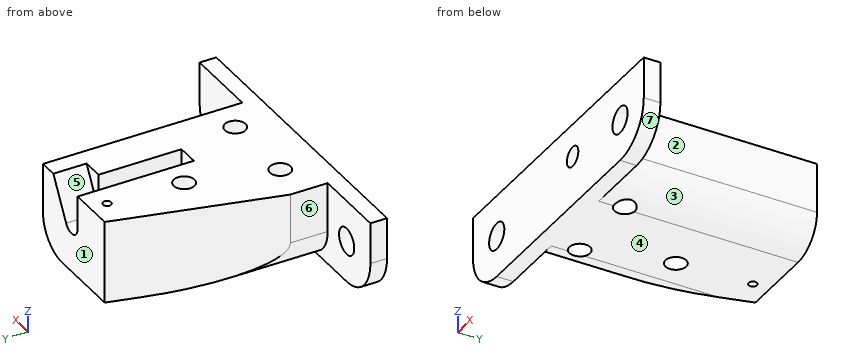
```python
from build123d import *

# Parameters (mm, degrees)
SKETCH1_R           = 1.6
BOSS_EXTRUDE1_DEPTH = 2
BOSS_EXTRUDE2_DEPTH = 26
CUT_EXTRUDE1_REACH  = 28
SKETCH3_R           = 1.2
CUT_EXTRUDE2_DEPTH  = 4
CUT_EXTRUDE3_DEPTH  = 14
CUT_EXTRUDE4_REACH  = 12
SKETCH6_R           = 0.5
SKETCH6_R_2         = 1.25


with BuildPart() as part:
    # Sketch1 → Boss-Extrude1 (new body)
    with BuildSketch(Plane(origin=(0, 0, 0), x_dir=(1, 0, 0), z_dir=(0, 1, 0))):
        with BuildLine():
            Line((0, 0), (36, 0))
            Line((36, 0), (36, 5))
            ThreePointArc((36, 5), (34.535533906, 8.535533906), (31, 10))
            Line((31, 10), (27, 10))
            Line((27, 10), (9, 10))
            Line((9, 10), (5, 10))
            ThreePointArc((5, 10), (1.464466094, 8.535533906), (0, 5))
            Line((0, 5), (0, 0))
        make_face()
        with Locations((5, 5)):
            Circle(SKETCH1_R, mode=Mode.SUBTRACT)
        with Locations((31, 5)):
            Circle(SKETCH1_R, mode=Mode.SUBTRACT)
    extrude(amount=BOSS_EXTRUDE1_DEPTH)

    # Sketch2 → Boss-Extrude2 (add)
    with BuildSketch(Plane(origin=(0, 0, 0), x_dir=(1, 0, 0), z_dir=(0, 1, 0))):
        with BuildLine():
            Line((27, 0), (27, 6))
            ThreePointArc((27, 6), (25.828427125, 8.828427125), (23, 10))
            Line((23, 10), (13, 10))
            ThreePointArc((13, 10), (10.171572875, 8.828427125), (9, 6))
            Line((9, 6), (9, 0))
            Line((9, 0), (27, 0))
        make_face()
    extrude(amount=BOSS_EXTRUDE2_DEPTH)

    # Sketch3 → Cut-Extrude1 (cut, up to next)
    with BuildSketch(Plane(origin=(0, 26, 0), x_dir=(1, 0, 0), z_dir=(0, 1, 0)), mode=Mode.PRIVATE) as cut_extrude1_sk1:
        with Locations((21, 4)):
            Circle(SKETCH3_R)
    cut_extrude1_tool1 = extrude(cut_extrude1_sk1.sketch, amount=-CUT_EXTRUDE1_REACH, mode=Mode.PRIVATE) & part.part
    add(cut_extrude1_tool1.solids().sort_by_distance((21, 26, -4))[0], mode=Mode.SUBTRACT)

    # Sketch4 → Cut-Extrude2 (cut)
    with BuildSketch(Plane(origin=(0, 26, 0), x_dir=(1, 0, 0), z_dir=(0, 1, 0))):
        with BuildLine():
            Line((22.125833025, 4.65), (24.810511777, 0))
            Line((24.810511777, 0), (19.7, 0))
            Line((19.7, 0), (19.7, 4))
            ThreePointArc((19.7, 4), (20.663535241, 5.255703574), (22.125833025, 4.65))
        make_face()
    extrude(amount=-CUT_EXTRUDE2_DEPTH, mode=Mode.SUBTRACT)

    # Sketch5 → Cut-Extrude3 (cut)
    with BuildSketch(Plane(origin=(0, 26, 0), x_dir=(1, 0, 0), z_dir=(0, 1, 0))):
        with BuildLine():
            Line((19.7, 4), (19.7, 0))
            Line((19.7, 0), (22.3, 0))
            Line((22.3, 0), (22.3, 4))
            ThreePointArc((22.3, 4), (21, 5.3), (19.7, 4))
        make_face()
    extrude(amount=-CUT_EXTRUDE3_DEPTH, mode=Mode.SUBTRACT)

    # Sketch6 → Cut-Extrude4 (cut, up to next)
    with BuildSketch(Plane.XY, mode=Mode.PRIVATE) as cut_extrude4_sk1:
        with Locations((17, 24)):
            Circle(SKETCH6_R)
    cut_extrude4_tool1 = extrude(cut_extrude4_sk1.sketch, amount=-CUT_EXTRUDE4_REACH, mode=Mode.PRIVATE) & part.part
    add(cut_extrude4_tool1.solids().sort_by_distance((17, 24, 0))[0], mode=Mode.SUBTRACT)
    # Sketch6 → Cut-Extrude4 (cut, up to next)
    with BuildSketch(Plane.XY, mode=Mode.PRIVATE) as cut_extrude4_sk2:
        with Locations((16.5, 15)):
            Circle(SKETCH6_R_2)
    cut_extrude4_tool2 = extrude(cut_extrude4_sk2.sketch, amount=-CUT_EXTRUDE4_REACH, mode=Mode.PRIVATE) & part.part
    add(cut_extrude4_tool2.solids().sort_by_distance((16.5, 15, 0))[0], mode=Mode.SUBTRACT)
    # Sketch6 → Cut-Extrude4 (cut, up to next)
    with BuildSketch(Plane.XY, mode=Mode.PRIVATE) as cut_extrude4_sk3:
        with Locations((13.75, 5)):
            Circle(SKETCH6_R_2)
    cut_extrude4_tool3 = extrude(cut_extrude4_sk3.sketch, amount=-CUT_EXTRUDE4_REACH, mode=Mode.PRIVATE) & part.part
    add(cut_extrude4_tool3.solids().sort_by_distance((13.75, 5, 0))[0], mode=Mode.SUBTRACT)
    # Sketch6 → Cut-Extrude4 (cut, up to next)
    with BuildSketch(Plane.XY, mode=Mode.PRIVATE) as cut_extrude4_sk4:
        with Locations((23.25, 5)):
            Circle(SKETCH6_R_2)
    cut_extrude4_tool4 = extrude(cut_extrude4_sk4.sketch, amount=-CUT_EXTRUDE4_REACH, mode=Mode.PRIVATE) & part.part
    add(cut_extrude4_tool4.solids().sort_by_distance((23.25, 5, 0))[0], mode=Mode.SUBTRACT)
    # Sketch6 → Cut-Extrude4 (cut, up to next)
    with BuildSketch(Plane.XY, mode=Mode.PRIVATE) as cut_extrude4_sk5:
        Polygon((9, 6.5), (14, 26), (9, 26), align=None)
    cut_extrude4_tool5 = extrude(cut_extrude4_sk5.sketch, amount=-CUT_EXTRUDE4_REACH, mode=Mode.PRIVATE) & part.part
    add(cut_extrude4_tool5.solids().sort_by_distance((10.666667, 19.5, 0))[0], mode=Mode.SUBTRACT)


solid = part.part
```
For this review, take the finished solid that the model builds, in its own axes (mm). Face numbers are marked on the shaded views. A direction names the side the tool comes from. Round coordinates to 2 decimals unless told otherwise and drop trailing zeros. Order: outer loops, then holes, each group sorted by start corner. A loop starts at its lowest first (then second) coordinate and runs counter-clockwise, first axis right, second up. Notation, with made-up numbers: (74, 31) -> (85, 31) arc R28 ccw to (85, 56) -> close; hole circle Ø11 at (-11.75, 3). An arc over 180 degrees is marked (long way). Use a Markdown table: item, result.
Item 1: Take a section at B-B (z = -1.25). State the section outline as (x, y) points, plus the area to 3 significant figures.
Resolved:
| item | result |
|---|---|
| outline | (0, 0) -> (36, 0) -> (36, 2) -> (27, 2) -> (27, 26) -> (24.09, 26) -> (24.09, 22) -> (22.3, 22) -> (22.3, 12) -> (19.7, 12) -> (19.7, 26) -> (14, 26) -> (9, 6.5) -> (9, 2) -> (0, 2) -> close; hole circle Ø2.5 at (13.75, 5); hole circle Ø2.5 at (16.5, 15); hole circle Ø1 at (17, 24); hole circle Ø2.5 at (23.25, 5) |
| area | 396 mm² |
Item 2: Take a section at D-D (y = 15). State the section outline as (x, z) points, plus the area to 3 significant figures.
Resolved:
| item | result |
|---|---|
| outline | (11.18, -9.56) arc R4 ccw to (13, -10) -> (15.25, -10) -> (15.25, 0) -> (11.18, 0) -> close; (17.75, -10) -> (23, -10) arc R4 ccw to (27, -6) -> (27, 0) -> (22.3, 0) -> (22.3, -4) arc R1.3 cw to (19.7, -4) -> (19.7, 0) -> (17.75, 0) -> close |
| area | 116 mm² |
Item 3: Take a section at C-C (x = 17). State the section outline as (y, z) points.
Resolved:
| item | result |
|---|---|
| outline | (0, -10) -> (13.85, -10) -> (13.85, 0) -> (0, 0) -> close; (16.15, -10) -> (23.5, -10) -> (23.5, 0) -> (16.15, 0) -> close; (24.5, -10) -> (26, -10) -> (26, 0) -> (24.5, 0) -> close |
Item 4: Take a section at A-A (y = 7). State the section outline as (x, z) points, plus the area to 3 significant figures.
Resolved:
| item | result |
|---|---|
| outline | (9.13, -7) arc R4 ccw to (13, -10) -> (23, -10) arc R4 ccw to (27, -6) -> (27, 0) -> (9.13, 0) -> close; hole circle Ø2.4 at (21, -4) |
| area | 168 mm² |
Item 5: For line 1 along Y through (x, z) = (17, -0.75); line 2 along X through (y, z) = (4.5, -5.5); line 3 along X through (y, z) = (5, -3), list the stretches that pass through material, from the lowest coordinate up. Write a range as [from, to].
Resolved:
| item | result |
|---|---|
| line 1 | y = [0, 13.85], [16.15, 23.5], [24.5, 26] |
| line 2 | x = [9, 12.6], [14.9, 22.1], [24.4, 27] |
| line 3 | x = [9, 12.5], [15, 20.34], [21.66, 22], [24.5, 27] |
Item 6: Draft analysis for pull direction X (two halves, no side actions). For the marked faces 4, 5, 6 and 7, state which applies: +X half, -X half, draft (parallel to the pull), parting line (faces both ways), or undercut.
Resolved:
| item | result |
|---|---|
| face 4 | draft |
| face 5 | undercut |
| face 6 | -X half |
| face 7 | +X half |
Item 7: Machinability: for the marked faces 1, 2 and 3, which of the approach directions +Z, -Z, +X, -X, +Y, -Y give a long, thin tool a straight path to every point of the face, cutting with its end or side? Answer none if there is none.
Resolved:
| item | result |
|---|---|
| face 1 | +Z, -Z, +X, -X, +Y |
| face 2 | +Z, -Z, +X, +Y |
| face 3 | -Z, +X, +Y |
Item 8: For pin 1 (2 mm diameter, centred on x = 16.5, y = 15, fed in from -Z); pin 2 (1 mm diameter, centred on y = 10.5, z = -7, fed in from +X); pin 3 (1.5 mm diameter, centred on x = 10, y = 4, fed in from -Z); pin 4 (1.2 mm diameter, centred on y = 15, z = -2, fed in from -X), all flat-tipped, find the tip position at first contact; note any pin that passes through.
Resolved:
| item | result |
|---|---|
| pin 1 | passes through |
| pin 2 | stops at x = 26.97 |
| pin 3 | stops at z = -9.31 |
| pin 4 | stops at x = 11.03 |
